```python
from build123d import *

# Parameters (mm, degrees)
F0_W     = 63.5
F0_H     = 88.9
F1_DEPTH = 6.35
F2_R     = 30.226
F3_DEPTH = 6.351
F4_W     = 49.529999
F4_H     = 51.943
F5_DEPTH = 6.351
F6_R     = 5.08


with BuildPart() as f1:
    # F0 (on Front) → F1 (new body)
    with BuildSketch(Plane.XZ):
        Rectangle(F0_W, F0_H)
    extrude(amount=F1_DEPTH)

    # F2 (on face) → F3 (cut, through all)
    with BuildSketch(Plane.XZ.offset(6.35)):
        with Locations((0, 44.45)):
            Circle(F2_R)
    extrude(amount=-F3_DEPTH, mode=Mode.SUBTRACT)

    # F4 (on face) → F5 (cut, through all)
    with BuildSketch(Plane.XZ.offset(6.35)):
        with Locations((-1e-06, -18.4785)):
            Rectangle(F4_W, F4_H)
    extrude(amount=-F5_DEPTH, mode=Mode.SUBTRACT)

    # F6
    f6_edges = [f1.edges().sort_by_distance(p)[0] for p in [
        (-24.765, -3.175, 7.493),
        (24.764999, -3.175, 7.493),
    ]]
    fillet(f6_edges, radius=F6_R)


solid = f1.part
```
Geometry: final body of the model. Coordinates: model frame, mm. A direction names the side the tool comes from. Coordinates: 2 decimals unless noted, no trailing zeros. Order: outer loops, then holes, each group sorted by start corner. A loop starts at its lowest first (then second) coordinate and runs counter-clockwise, first axis right, second up. Notation, with made-up numbers: (-4, 59) -> (26, 59) arc R22 cw to (26, 80) -> close; hole circle Ø3 at (85.5, -17). An arc over 180 degrees is marked (long way). Answer in a Markdown table with one row per item.
Item 1: Section D-D on z = 18.5. Output: boundary loops of the cut face in (x, y), plus the area to 3 significant figures.
Return value:
| item | result |
|---|---|
| outline | (-31.75, -6.35) -> (-15.5, -6.35) -> (-15.5, 0) -> (-31.75, 0) -> close; (15.5, -6.35) -> (31.75, -6.35) -> (31.75, 0) -> (15.5, 0) -> close |
| area | 206 mm² |
Item 2: Draft query along X for faces 3 (the flat face through (28, -3, -44.45)), 4 (the flat face through (31.75, -3, -1)), 5 (the flat face through (0, -3, 7.493)). Return one class per face: released by +X, released by -X, zero draft, split by the parting line, or undercut.
Return value:
| item | result |
|---|---|
| face 3 | zero draft |
| face 4 | released by +X |
| face 5 | undercut |
Item 3: Section B-B on y = -1.5. Output: boundary loops of the cut face in (x, z) (3 decimals).
Return value:
| item | result |
|---|---|
| outline | (-31.75, -44.45) -> (-24.765, -44.45) -> (-24.765, 2.413) arc R5.08 cw to (-19.685, 7.493) -> (19.685, 7.493) arc R5.08 cw to (24.765, 2.413) -> (24.765, -44.45) -> (31.75, -44.45) -> (31.75, 44.45) -> (30.226, 44.45) arc R30.226 cw to (-30.226, 44.45) -> (-31.75, 44.45) -> close |
Item 4: Section A-A on z = -34. Output: boundary loops of the cut face in (x, y) (3 decimals), plus the area to 3 significant figures.
Return value:
| item | result |
|---|---|
| outline | (-31.75, -6.35) -> (-24.765, -6.35) -> (-24.765, 0) -> (-31.75, 0) -> close; (24.765, -6.35) -> (31.75, -6.35) -> (31.75, 0) -> (24.765, 0) -> close |
| area | 88.7 mm² |
Item 5: Access query for faces 1 (the flat face through (-7, 0, 10)), 2 (the cylindrical face through (23.316, -3.131, 5.965)). Directions: +Z, -Z, +X, -X, +Y, -Y. A direction counts if a zero-diameter tool reaches every point of the face in a straight line with its end or side. Return the directions, or none.
Return value:
| item | result |
|---|---|
| face 1 | +Z, -Z, +X, -X, +Y |
| face 2 | -Z, +Y, -Y |
Item 6: Ray query, L1, parallel to X at y = -2.25, z = -22 (3 decimals); L2, parallel to Z at x = 1, y = -5.5; L3, parallel to X at y = -5.25, z = 40. Return the intervals inside material, ascending.
Return value:
| item | result |
|---|---|
| L1 | x = -31.75 to -24.765, 24.765 to 31.75 |
| L2 | z = 7.49 to 14.24 |
| L3 | x = -31.75 to -29.9, 29.9 to 31.75 |
Item 7: Section C-C on x = 0. Output: boundary loops of the cut face in (y, z).
Return value:
| item | result |
|---|---|
| outline | (-6.35, 7.49) -> (0, 7.49) -> (0, 14.22) -> (-6.35, 14.22) -> close |
Item 8: Contact query for a flat-ended pin moving along its axis: P1, Ø1, axis at x = -10.5, y = -5, coming from the -Z side. Output: stop coordinate, or through.
Return value:
| item | result |
|---|---|
| P1 | stops at z = 7.49 |
